from build123d import *

# Parameters (mm, degrees)
SKETCH1_W               = 250
SKETCH1_H               = 250
BOSS_EXTRUDE1_DEPTH     = 7
CUT_EXTRUDE2_DEPTH      = 4
CUT_EXTRUDE3_DEPTH      = 177.91523394
CUT_EXTRUDE4_DEPTH      = 177.91523394
CUT_EXTRUDE5_DEPTH      = 2.3
CIRPATTERN1_COUNT       = 4
SKETCH8_R               = 5
CUT_EXTRUDE6_DEPTH      = 177.91523394
SKETCH9_R               = 1.5
CUT_EXTRUDE7_DEPTH      = 177.821944339
SKETCH10_R              = 2.8
CUT_EXTRUDE8_DEPTH      = 1.6
SKETCH13_R              = 1.5
CUT_EXTRUDE11_DEPTH     = 177.91523394
LPATTERN1_COUNT         = 2
LPATTERN1_PITCH         = 50
LPATTERN1_COUNT_DIR2    = 2
LPATTERN1_PITCH_DIR2    = 29
SKETCH14_R              = 1.5
CUT_EXTRUDE12_DEPTH     = 10
MIRROR3_COPY_1_SKETCH_R = 1.5
MIRROR3_COPY_1_DEPTH    = 10


with BuildPart() as part:
    # Sketch1 → Boss-Extrude1 (new body)
    with BuildSketch(Plane(origin=(0, 0, 0), x_dir=(1, 0, 0), z_dir=(0, 1, 0))):
        Rectangle(SKETCH1_W, SKETCH1_H)
    extrude(amount=BOSS_EXTRUDE1_DEPTH)

    # Sketch4 → Cut-Extrude2 (cut)
    with BuildSketch(Plane(origin=(0, 7, 0), x_dir=(1, 0, 0), z_dir=(0, 1, 0))):
        with BuildLine():
            ThreePointArc((-29.508381723, 43.240928622), (-39.076271632, 39.076271632), (-43.240928622, 29.508381723))
            ThreePointArc((-43.240928622, 29.508381723), (-52.35, 0), (-43.240928622, -29.508381723))
            ThreePointArc((-43.240928622, -29.508381723), (-39.076271632, -39.076271632), (-29.508381723, -43.240928622))
            ThreePointArc((-29.508381723, -43.240928622), (0, -52.35), (29.508381723, -43.240928622))
            ThreePointArc((29.508381723, -43.240928622), (39.076271632, -39.076271632), (43.240928622, -29.508381723))
            ThreePointArc((43.240928622, -29.508381723), (52.35, 0), (43.240928622, 29.508381723))
            ThreePointArc((43.240928622, 29.508381723), (39.076271632, 39.076271632), (29.508381723, 43.240928622))
            ThreePointArc((29.508381723, 43.240928622), (0, 52.35), (-29.508381723, 43.240928622))
        make_face()
    extrude(amount=-CUT_EXTRUDE2_DEPTH, mode=Mode.SUBTRACT)

    # Sketch5 → Cut-Extrude3 (cut, through all)
    with BuildSketch(Plane(origin=(0, 7, 0), x_dir=(1, 0, 0), z_dir=(0, 1, 0))):
        Polygon((-40.2277855, 40.2277855), (-38.35395253, 42.10161847), (-73.709291589, 77.456957529), (-77.456957529, 73.709291589), (-42.10161847, 38.35395253), align=None)
    cut_extrude3 = extrude(amount=-CUT_EXTRUDE3_DEPTH, mode=Mode.SUBTRACT)

    # Sketch6 → Cut-Extrude4 (cut, through all)
    with BuildSketch(Plane(origin=(0, 7, 0), x_dir=(1, 0, 0), z_dir=(0, 1, 0))):
        Polygon((-26.542386103, 45.987822586), (-61.897725163, 81.343161645), (-59.493562107, 83.747324701), (-24.138223047, 48.391985642), align=None)
        Polygon((-81.343161645, 61.897725163), (-83.747324701, 59.493562107), (-48.391985642, 24.138223047), (-45.987822586, 26.542386103), align=None)
    cut_extrude4 = extrude(amount=-CUT_EXTRUDE4_DEPTH, mode=Mode.SUBTRACT)

    # Sketch7 → Cut-Extrude5 (cut)
    with BuildSketch(Plane.XZ):
        Polygon((-90.835333565, -74.571877598), (-41.337858882, -25.074402915), (-25.074402915, -41.337858882), (-74.571877598, -90.835333565), align=None)
    cut_extrude5 = extrude(amount=-CUT_EXTRUDE5_DEPTH, mode=Mode.SUBTRACT)

    # CirPattern1: Cut-Extrude3, Cut-Extrude4, Cut-Extrude5 ×4 about axis
    cirpattern1_axis = Axis((0, 0, 0), (0, 1, 0))
    add([cut_extrude3.rotate(cirpattern1_axis, i * 360 / CIRPATTERN1_COUNT) for i in range(1, CIRPATTERN1_COUNT)], mode=Mode.SUBTRACT)
    add([cut_extrude4.rotate(cirpattern1_axis, i * 360 / CIRPATTERN1_COUNT) for i in range(1, CIRPATTERN1_COUNT)], mode=Mode.SUBTRACT)
    add([cut_extrude5.rotate(cirpattern1_axis, i * 360 / CIRPATTERN1_COUNT) for i in range(1, CIRPATTERN1_COUNT)], mode=Mode.SUBTRACT)

    # Sketch8 → Cut-Extrude6 (cut, through all)
    with BuildSketch(Plane(origin=(0, 7, 0), x_dir=(1, 0, 0), z_dir=(0, 1, 0))):
        with Locations(Location((14.5, 14.5, 0), (0, 0, 270))):
            Circle(SKETCH8_R)
        with Locations(Location((-14.5, 14.5, 0), (0, 0, 270))):
            Circle(SKETCH8_R)
        with Locations(Location((-14.5, -14.5, 0), (0, 0, 270))):
            Circle(SKETCH8_R)
        with Locations(Location((14.5, -14.5, 0), (0, 0, 270))):
            Circle(SKETCH8_R)
    extrude(amount=-CUT_EXTRUDE6_DEPTH, mode=Mode.SUBTRACT)

    # Sketch9 → Cut-Extrude7 (cut, through all)
    with BuildSketch(Plane(origin=(0, 3, 0), x_dir=(1, 0, 0), z_dir=(0, 1, 0))):
        with Locations(Location((-15.6, -30, 0), (0, 0, 270))):
            Circle(SKETCH9_R)
        with Locations(Location((15.9, -30, 0), (0, 0, 90))):
            Circle(SKETCH9_R)
    cut_extrude7 = extrude(amount=-CUT_EXTRUDE7_DEPTH, mode=Mode.SUBTRACT)

    # Sketch10 → Cut-Extrude8 (cut)
    with BuildSketch(Plane(origin=(0, 3, 0), x_dir=(1, 0, 0), z_dir=(0, 1, 0))):
        with Locations(Location((-15.6, -30, 0), (0, 0, 270))):
            Circle(SKETCH10_R)
        with Locations(Location((15.9, -30, 0), (0, 0, 270))):
            Circle(SKETCH10_R)
    cut_extrude8 = extrude(amount=-CUT_EXTRUDE8_DEPTH, mode=Mode.SUBTRACT)

    # Sketch13 → Cut-Extrude11 (cut, through all)
    with BuildSketch(Plane(origin=(0, 7, 0), x_dir=(1, 0, 0), z_dir=(0, 1, 0))):
        with Locations(Location((25.15, 120, 0), (0, 0, 270))):
            Circle(SKETCH13_R)
    cut_extrude11 = extrude(amount=-CUT_EXTRUDE11_DEPTH, mode=Mode.SUBTRACT)

    # LPattern1: Cut-Extrude11 2 × 2
    with Locations(*[(-i * LPATTERN1_PITCH, 0, j * LPATTERN1_PITCH_DIR2) for i in range(LPATTERN1_COUNT) for j in range(LPATTERN1_COUNT_DIR2) if (i, j) != (0, 0)]):
        add(cut_extrude11, mode=Mode.SUBTRACT)

    # Mirror1: Cut-Extrude7, Cut-Extrude8 across plane
    add(cut_extrude7.mirror(Plane.XY), mode=Mode.SUBTRACT)
    add(cut_extrude8.mirror(Plane.XY), mode=Mode.SUBTRACT)

    # Sketch14 → Cut-Extrude12 (cut)
    with BuildSketch(Plane(origin=(0, 7, 0), x_dir=(1, 0, 0), z_dir=(0, 1, 0))):
        with Locations(Location((120, -100, 0), (0, 0, 270))):
            Circle(SKETCH14_R)
        with Locations(Location((120, -120, 0), (0, 0, 270))):
            Circle(SKETCH14_R)
        with Locations(Location((100, -120, 0), (0, 0, 270))):
            Circle(SKETCH14_R)
    cut_extrude12 = extrude(amount=-CUT_EXTRUDE12_DEPTH, mode=Mode.SUBTRACT)

    # Mirror2: Cut-Extrude12 across plane
    add(cut_extrude12.mirror(Plane(origin=(0, 0, 0), x_dir=(0, 0, 1), z_dir=(1, 0, 0))), mode=Mode.SUBTRACT)

    # Mirror3: Cut-Extrude12 across plane
    add(cut_extrude12.mirror(Plane.XY), mode=Mode.SUBTRACT)

    # Mirror3 copy 1 sketch → Mirror3 copy 1 (cut)
    with BuildSketch(Plane(origin=(0, 7, 0), x_dir=(-1, 0, 0), z_dir=(0, 1, 0))):
        with Locations(Location((120, -100, 0), (0, 0, 270))):
            Circle(MIRROR3_COPY_1_SKETCH_R)
        with Locations(Location((120, -120, 0), (0, 0, 270))):
            Circle(MIRROR3_COPY_1_SKETCH_R)
        with Locations(Location((100, -120, 0), (0, 0, 270))):
            Circle(MIRROR3_COPY_1_SKETCH_R)
    extrude(amount=-MIRROR3_COPY_1_DEPTH, mode=Mode.SUBTRACT)


solid = part.part
The model under review builds one solid part; all positions refer to its coordinate system, in mm. A direction names the side the tool comes from. Round coordinates to 2 decimals unless told otherwise and drop trailing zeros. Loops run counter-clockwise (first coordinate to the right, second up) from the corner with the lowest first, then second, coordinate; pieces in that order, holes last. Notation, with made-up numbers: (86.25, -18.75) -> (136.25, -18.75) arc R28 ccw to (136.25, 20.25) -> close; hole circle Ø6 at (51.25, 48.25). An arc over 180 degrees is marked (long way). Write item = value, one per line. Start each with the question number.
Item 1: To check wall thickness, follow L1, parallel to X at y = 4.5, z = -91; L2, parallel to Z at x = -120, y = 1.75; L3, parallel to Z at x = -67, y = 5. State the ranges of each line that lie inside material, in increasing order.
Item 2: Take a section at A-A on x = -67. Give the boundary of the cut face in (y, z), plus the area to 3 significant figures.
Item 3: Take a section at B-B on z = 14.5. Give the boundary of the cut face in (x, y), plus the area to 3 significant figures.
Item 4: Take a section at C-C on z = 56. Count the separate pieces of the cut face and the enclosed holes in it, plus the area to 3 significant figures.
Item 5: Mouldability with a two-part tool opening along X and no side actions: class faces 4 (the flat face through (-60, 2.3, -55)), 5 (the flat face through (-33.32, 1.13, -33.09)) as released by +X, released by -X, zero draft, split by the parting line, or undercut.
Item 6: Insertion check: pin 1 (13 mm diameter, centred on x = -14.5, z = -14.5, fed in from +Y); pin 2 (19.5 mm diameter, centred on x = -67.5, z = 67, fed in from -Y); pin 3 (5 mm diameter, centred on x = 15.9, z = -30, fed in from +Y). Each pin has a flat end and moves straight along its axis. Give the tip position at first contact, or say it passes through.
Item 7: For faces 1 (the flat face through (66.317, 3.549, -42.063)), 2 (the flat face through (82.59, 1.13, 82.82)), 3 (the cylindrical face through (0.44, 5.03, -52.35)), list the 3-axis set-ups (+Z, -Z, +X, -X, +Y, -Y) from which the entire face can be reached by the end or side of a thin tool; tool diameter is ignored.
Result:
q1.L1 = -125 to -26.35, -23.35 to 23.65, 26.65 to 125
q1.L2 = -125 to -121.5, -118.5 to -101.5, -98.5 to 98.5, 101.5 to 118.5, 121.5 to 125
q1.L3 = -125 to -70.75, -63.25 to -47.55, -42.75 to 42.75, 47.55 to 63.25, 70.75 to 125
q2.outline = (0, -125) -> (7, -125) -> (7, -70.75) -> (2.3, -70.75) -> (2.3, -83.26) -> (0, -83.26) -> close; (0, -50.74) -> (2.3, -50.74) -> (2.3, -63.25) -> (7, -63.25) -> (7, -47.55) -> (0, -47.55) -> close; (0, -42.75) -> (7, -42.75) -> (7, 42.75) -> (0, 42.75) -> close; (0, 47.55) -> (7, 47.55) -> (7, 63.25) -> (2.3, 63.25) -> (2.3, 50.74) -> (0, 50.74) -> close; (0, 83.26) -> (2.3, 83.26) -> (2.3, 70.75) -> (7, 70.75) -> (7, 125) -> (0, 125) -> close
q2.area = 1,460 mm²
q3.outline = (-125, 0) -> (-19.5, 0) -> (-19.5, 3) -> (-50.3, 3) -> (-50.3, 7) -> (-125, 7) -> close; (-9.5, 0) -> (9.5, 0) -> (9.5, 3) -> (-9.5, 3) -> close; (19.5, 0) -> (125, 0) -> (125, 7) -> (50.3, 7) -> (50.3, 3) -> (19.5, 3) -> close
q3.area = 1,290 mm²
q4.separate_pieces = 7
q4.enclosed_holes = 0
q4.area = 1,400 mm²
q5.face_4 = undercut
q5.face_5 = undercut
q6.pin_1 = 3
q6.pin_2 = 2.3
q6.pin_3 = 1.4
q7.face_1 = +Y, -Y
q7.face_2 = -Y
q7.face_3 = +Y
